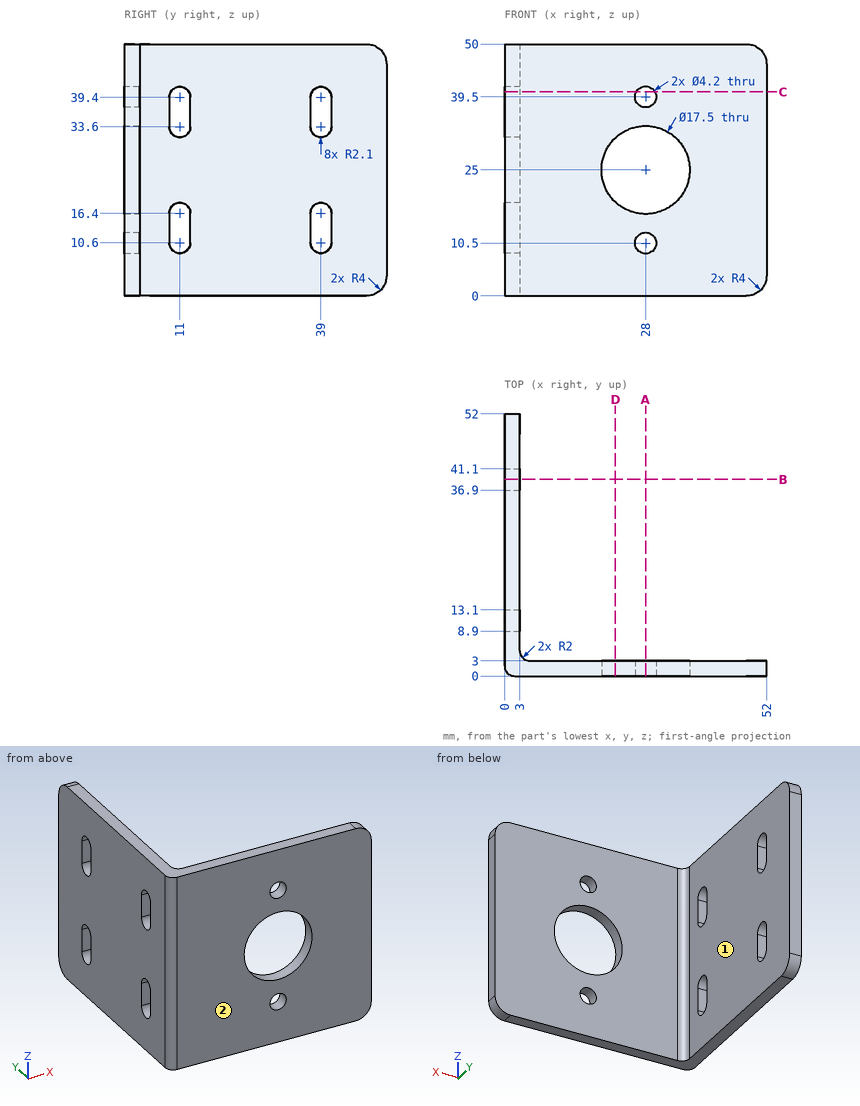
Part print with two shaded views. Sizes in mm from the minimum x, y, z corner. A direction names the side the tool comes from. Round coordinates to 2 decimals unless told otherwise and drop trailing zeros. Loops run counter-clockwise (first coordinate to the right, second up) from the corner with the lowest first, then second, coordinate; pieces in that order, holes last. Notation, with made-up numbers: M 30,-27.75 L 75,-27.75 A14 cw 75,-8.75 Z; hole C 40,83 d9. An arc over 180 degrees is marked long. Put each result on its own line as item: value. Start each with the question number.
Item 1: Cut at D-D (x = 22). List the corners of the cut face in (y, z).
Item 2: 3-axis set-ups, long thin cutter, end or side, ignore diameter. For the marked faces 1 and 2: which of +Z, -Z, +X, -X, +Y, -Y reach the whole face in a straight line?
Item 3: Drill centre lines: line 1 along X through (y, z) = (1.75, 10.5); line 2 along Y through (x, z) = (37.5, 18.5). Where is each one in solid material? Low to high.
Item 4: Cut at C-C (z = 40.5). List the corners of the cut face in (x, y).
Item 5: Drop flat-ended pins along their axis: P1, Ø3, axis at y = 19, z = 23, coming from the +X side; P2, Ø0.9, axis at x = 1, z = 36, coming from the -Y side. Give the stop position or say it passes through.
Item 6: Cut at A-A (x = 28). List the corners of the cut face in (y, z).
Item 7: Cut at B-B (y = 39). List the corners of the cut face in (x, z).
Answer block:
1. outline: M 0,0 L 3,0 L 3,18.63 L 0,18.63 Z; M 0,31.37 L 3,31.37 L 3,50 L 0,50 Z
2. face 1: +Z, -Z, +X, +Y
2. face 2: +Z, -Z, +X, -X, -Y
3. line 1: 0.02 to 25.9, 30.1 to 52
3. line 2: 0 to 3
4. outline: M 0,2 A2 ccw 2,0 L 26.15,0 L 26.15,3 L 5,3 A2 cw 3,5 L 3,9.21 L 0,9.21 Z; M 0,12.79 L 3,12.79 L 3,37.21 L 0,37.21 Z; M 0,40.79 L 3,40.79 L 3,52 L 0,52 Z; M 29.85,0 L 52,0 L 52,3 L 29.85,3 Z
5. P1: x = 3
5. P2: y = 0.08
6. outline: M 0,0 L 3,0 L 3,8.4 L 0,8.4 Z; M 0,12.6 L 3,12.6 L 3,16.25 L 0,16.25 Z; M 0,33.75 L 3,33.75 L 3,37.4 L 0,37.4 Z; M 0,41.6 L 3,41.6 L 3,50 L 0,50 Z
7. outline: M 0,0 L 3,0 L 3,8.5 L 0,8.5 Z; M 0,18.5 L 3,18.5 L 3,31.5 L 0,31.5 Z; M 0,41.5 L 3,41.5 L 3,50 L 0,50 Z
